Read the model definition and answer for the solid it produces. Units are mm, in the model's axes. Round coordinates to 2 decimals unless told otherwise and drop trailing zeros. Write each loop counter-clockwise with the first axis right and the second up, starting at its lowest first coordinate (ties: lowest second). Pieces come first, ordered by that corner, then holes.
from build123d import *

# Parameters (mm, degrees)
F0_W     = 65
F0_H     = 45
F0_W_2   = 60.5
F0_H_2   = 40.5
F1_DEPTH = 2
F0_W_3   = 52
F0_H_3   = 32
F2_DEPTH = 4
F3_R     = 3


with BuildPart() as f1:
    # F0 (on Top) → F1 (new body)
    with BuildSketch(Plane.XY):
        Rectangle(F0_W, F0_H)
        Rectangle(F0_W_2, F0_H_2, mode=Mode.SUBTRACT)
    extrude(amount=F1_DEPTH)

    # F0 (on Top) → F2 (join)
    with BuildSketch(Plane.XY):
        Rectangle(F0_W_2, F0_H_2)
        Rectangle(F0_W_3, F0_H_3, mode=Mode.SUBTRACT)
        Rectangle(F0_W_3, F0_H_3)
    extrude(amount=F2_DEPTH)

    # F3
    f3_edges = [f1.edges().sort_by_distance(p)[0] for p in [
        (-32.5, 22.5, 1),
        (32.5, 22.5, 1),
        (32.5, -22.5, 1),
        (-32.5, -22.5, 1),
    ]]
    fillet(f3_edges, radius=F3_R)


solid = f1.part
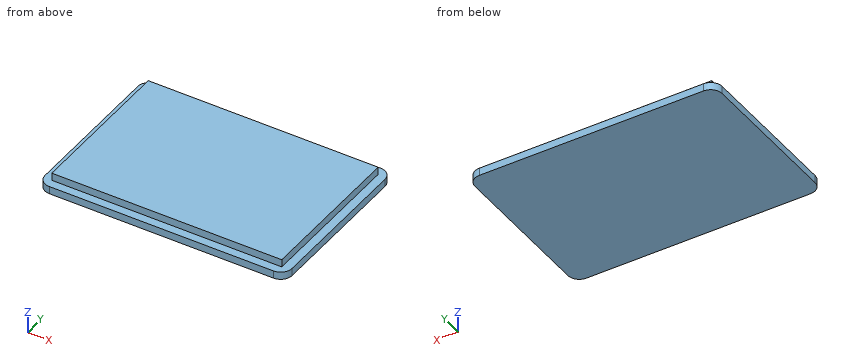
Q1. Section C-C (z = 3.2) is taken. Determine the outline of the cut face in (x, y), then the cut area to 3 significant figures.
Verdict:
outline: (-30.25, -20.25) - (30.25, -20.25) - (30.25, 20.25) - (-30.25, 20.25) - close
area: 2,450 mm2
Q2. Section A-A (y = -5) is taken. Determine the outline of the cut face in (x, z).
Verdict:
outline: (-32.5, 0) - (32.5, 0) - (32.5, 2) - (30.25, 2) - (30.25, 4) - (-30.25, 4) - (-30.25, 2) - (-32.5, 2) - close
Q3. Section B-B (x = 27) is taken. Determine the outline of the cut face in (y, z), then the cut area to 3 significant figures.
Verdict:
outline: (-22.5, 0) - (22.5, 0) - (22.5, 2) - (20.25, 2) - (20.25, 4) - (-20.25, 4) - (-20.25, 2) - (-22.5, 2) - close
area: 171 mm2
Q4. Straight lines are drawn through the part: probe 1 along X at (y, z) = (-12.5, 3.7); probe 2 along Y at (x, z) = (-13.5, 3.75); probe 3 along X at (y, z) = (20.5, 1.8). For each, find the intervals that lie inside material, in ascending order.
Verdict:
probe 1: x = -30.25 to 30.25
probe 2: y = -20.25 to 20.25
probe 3: x = -32.33 to 32.33
Q5. Flat-ended cylindrical pins translate along their axes: pin 1 Ø1.6 at (x, z) = (8, 3) entering from -Y; pin 2 Ø0.6 at (y, z) = (9.5, 3) entering from -X. Find the tip coordinate at first contact, or state that the pin passes through.
Verdict:
pin 1: stops at y = -20.25
pin 2: stops at x = -30.25
